```python
from build123d import *

# Parameters (mm, degrees)
SKETCH2_R                = 3.96875
BOSS_EXTRUDE1_DEPTH      = 2.4765
BOSS_EXTRUDE1_DEPTH_BACK = 2.4765
SKETCH4_R                = 3.96875
BOSS_EXTRUDE2_DEPTH      = 4.953
CUT_SWEEP1_PITCH         = 1.411111111
CUT_SWEEP1_HEIGHT        = 6.364111111
CUT_SWEEP1_RADIUS        = 3.96875
CUT_SWEEP1_START_ANGLE   = 180
SKETCH8_R                = 4.365625
BOSS_EXTRUDE3_DEPTH      = 4.953


with BuildPart() as part:
    # Sketch2 → Boss-Extrude1 (new, two sides)
    with BuildSketch(Plane(origin=(0, 0, 0), x_dir=(1, 0, 0), z_dir=(0, 1, 0))) as boss_extrude1_sk:
        Polygon((0, 7.332348419), (-6.35, 3.666174209), (-6.35, -3.666174209), (0, -7.332348419), (6.35, -3.666174209), (6.35, 3.666174209), align=None)
        with Locations(Location((0, 0, 0), (0, 0, 270))):
            Circle(SKETCH2_R, mode=Mode.SUBTRACT)
    extrude(amount=BOSS_EXTRUDE1_DEPTH)
    extrude(boss_extrude1_sk.sketch, amount=-BOSS_EXTRUDE1_DEPTH_BACK)

    # Sketch3 → Cut-Revolve1 (revolve, cut)
    with BuildSketch(Plane(origin=(0, 0, 0), x_dir=(0, 0, -1), z_dir=(1, 0, 0))):
        Polygon((-7.332348419, 1.909340876), (-6.35, 2.4765), (-7.332348419, 2.4765), align=None)
        Polygon((-7.332348419, -1.909340876), (-6.35, -2.4765), (-7.332348419, -2.4765), align=None)
        Polygon((-4.365625, 2.4765), (-3.96875, 2.4765), (-3.96875, 2.079625), align=None)
        Polygon((-4.365625, -2.4765), (-3.96875, -2.4765), (-3.96875, -2.079625), align=None)
    revolve(axis=Axis((0, 2.4765, 0), (0, -1, 0)), mode=Mode.SUBTRACT)

    # Sketch8 → Boss-Extrude3 (add)
    with BuildSketch(Plane(origin=(0, 2.4765, 0), x_dir=(1, 0, 0), z_dir=(0, 1, 0))):
        Circle(SKETCH8_R)
    extrude(amount=-BOSS_EXTRUDE3_DEPTH)


with BuildPart() as body_2:
    # Sketch4 → Boss-Extrude2 (new body)
    with BuildSketch(Plane(origin=(0, 2.4765, 0), x_dir=(1, 0, 0), z_dir=(0, 1, 0))):
        with Locations(Location((0, 0, 0), (0, 0, 270))):
            Circle(SKETCH4_R)
    extrude(amount=-BOSS_EXTRUDE2_DEPTH)

    # Cut-Sweep1: sweep along a helix
    with BuildLine() as cut_sweep1_path:
        add(Helix(CUT_SWEEP1_PITCH, CUT_SWEEP1_HEIGHT, CUT_SWEEP1_RADIUS, center=(0, 2.4765, 0), direction=(0, -1, 0), mode=Mode.PRIVATE).rotate(Axis((0, 2.4765, 0), (0, -1, 0)), CUT_SWEEP1_START_ANGLE))
    # Sketch6 → Cut-Sweep1 (sweep, cut)
    with BuildSketch(Plane(origin=(0, 0, 0), x_dir=(0, 0, -1), z_dir=(1, 0, 0))):
        Polygon((-4.045128629, 2.432402778), (-4.045128629, 3.755319444), (-3.052206448, 3.182055556), (-3.052206448, 3.005666667), align=None)
    sweep(path=cut_sweep1_path.line, is_frenet=True, mode=Mode.SUBTRACT)

    # Sketch7 → Revolve1 (revolve)
    with BuildSketch(Plane(origin=(0, 0, 0), x_dir=(0, 0, -1), z_dir=(1, 0, 0)), mode=Mode.PRIVATE) as revolve1_sk:
        Polygon((-4.365625, 2.4765), (-2.38125, 0.492125), (0, 0.492125), (0, 2.4765), align=None)
        Polygon((-4.365625, -2.4765), (0, -2.4765), (0, -0.492125), (-2.38125, -0.492125), align=None)
    revolve(revolve1_sk.sketch.rotate(Axis((0, -2.4765, 0), (0, 1, 0)), 303.531095579), axis=Axis((0, -2.4765, 0), (0, 1, 0)))


with BuildPart() as part_1:
    add(part.part)

    # Combine1: cut body 2
    add(body_2.part, mode=Mode.SUBTRACT)


solid = part_1.part
```
Can you work these out from the model? Positions are in its coordinate system, mm. Round coordinates to 2 decimals unless told otherwise and drop trailing zeros. Answer in a Markdown table with one row per item.
Item 1: If I drill on probe 1 along Z at (x, y) = (-0.5, -0.6); probe 2 along X at (y, z) = (0.3, -0.75); probe 3 along X at (y, z) = (-0.8, 0), over which ranges is the centre line in solid material (lowest first)?
Answer block:
| item | result |
|---|---|
| probe 1 | -7.04 to -3.21, 3.85 to 7.04 |
| probe 2 | -6.35 to -3.56, 3.46 to 6.35 |
| probe 3 | -6.35 to -3.97, 3.05 to 6.35 |
Item 2: Will these pins go through, and if not, where does the flat tip stop? P1, Ø1, axis at x = 4, y = -1, coming from the -Z side; P2, Ø1, axis at x = 2.5, y = -0.5, coming from the +Z side; P3, Ø1, axis at x = 1.5, y = 1, coming from the +Z side (3 decimals).
Answer block:
| item | result |
|---|---|
| P1 | z = -5.31 |
| P2 | z = 6.18 |
| P3 | z = 6.755 |
Item 3: Suppose I cut it at A-A, the plane x = 3.75. Give the number of separate pieces and of enclosed holes in the cut face, plus the area to 3 significant figures.
Answer block:
| item | result |
|---|---|
| separate pieces | 1 |
| enclosed holes | 3 |
| area | 44.9 mm² |
Item 4: We'd pull the mould along Y, two halves only. Please class faces 1 (the flat face through (3.131, 0.035, 5.525)), 2 (the conical face through (5.69, 2.34, -3.31)), 3 (the conical face through (-5.71, -2.34, -3.28)): released by +Y, released by -Y, zero draft, split by the parting line, or undercut.
Answer block:
| item | result |
|---|---|
| face 1 | zero draft |
| face 2 | released by +Y |
| face 3 | released by -Y |
